Autodesk Inventor part; units mm, degrees
ref_plane "Work Plane1" through (1.525, 0, 0) normal (0, 0, 1) x (1, 0, 0)
ref_plane "YZ Plane" through (0, 0, 0) normal (1, 0, 0) x (0, 1, 0)
ref_plane "XZ Plane" through (0, 0, 0) normal (0, 1, 0) x (-1, 0, 0)
sketch "Sketch1" plane through (0, 0, 0) normal (0, 0, 1) x (1, 0, 0)
  line L0 (0, 3.175) -> (38.1, 3.175)
  line L1 (38.1, 3.175) -> (38.1, 0)
  line L2 (38.1, 0) -> (0, 0)
  line L3 (-7.62, 0) -> (45.72, 0)
  line L4 (0, -0.635) -> (0, 3.81)
  line L5 (0, 3.175) -> (0, 0)
  dimension "d2" = 6.35
  dimension "d59" = 38.1
revolve "Body" add sketch "Sketch1" angle 360 about axis through (38.1, 0, 0) along (-1, 0, 0)
sketch "Sketch2" plane through (0, 0, 0) normal (-1, 0, 0) x (0, 0, 1)
  line L0 (0, 6.4231) -> (5.5626, 3.2116)
  line L1 (5.5626, 3.2116) -> (5.5626, -3.2116)
  line L2 (5.5626, -3.2116) -> (0, -6.4231)
  line L3 (0, -6.4231) -> (-5.5626, -3.2116)
  line L4 (-5.5626, -3.2116) -> (-5.5626, 3.2116)
  line L5 (-5.5626, 3.2116) -> (0, 6.4231)
  line L6 (-7.7876, 0) -> (7.7876, 0)
  line L7 (0, 8.9924) -> (0, -8.9924)
  point P0 (0, 0)
  point P1 (0, 0)
  dimension "d11" = 11.1252
extrude "Head" add sketch "Sketch2" along normal blind 4.826
sketch "Sketch4" plane through (0, 0, 0) normal (0, 0, 1) x (1, 0, 0)
  line L0 (-4.1837, 6.6751) -> (-4.826, 5.5626)
  line L1 (-1.1, 0) -> (-0.234, 0)
  line L2 (-5.7444, 0) -> (0.6844, 0)
  line L3 (-4.826, 6.6751) -> (-4.1837, 6.6751)
  line L4 (-4.826, 5.5626) -> (-4.826, 6.6751)
  line L5 (0, 8.0101) -> (0, -1.335)
  dimension "d65" = 11.1252
  dimension "d67" = 30
  dimension "d68" = 13.3502
  dimension "d69" = 4.826
revolve "Chamfer1" cut sketch "Sketch4" angle 360 about axis through (-1.1, 0, 0) along (1, 0, 0)
thread "Thread"
chamfer "Chamfer2" distance 0.635 distance2 0.6351 1 edges at (38.1, -3.175, 0) measured on face at (38.1, -0.8017, 1.6073)
fillet "Fillet" radius 0.0635 1 edges at (0, -3.175, 0)
ref_plane "Work Plane1" through (1.525, 0, 0) normal (0, 0, 1) x (1, 0, 0)
equation "\"d2\" = GD"
equation "\"d59\" = NLG"
equation "\"d11\" = SW"
equation "\"d3\" = KOH"
equation "\"d15\" = GEL"
equation "\"d6\" = -0.5 * SPD + 0.5 * GD"
equation "\"d71\" = RR"
equation "\"d65\" = SW"
equation "\"d67\" = ANG1"
equation "\"d68\" = 1.2 * SW"
equation "\"d69\" = KOH"
equation "\"NLG\" = 38.1"
equation "\"GD\" = NND"
equation "\"BDM\" = NND"
equation "\"KOH\" = 4.826"
equation "\"GEL\" = 32.385"
equation "\"SW\" = 11.1252"
equation "\"SW0\" = SW"
equation "\"SPD\" = GD1"
equation "\"SD2\" = NND"
equation "\"SD\" = 0"
equation "\"ANG1\" = 30deg"
equation "\"GAL\" = 0.635"
equation "\"GUL\" = GAL"
equation "\"RR\" = 0.0635"
equation "\"RR1\" = 0.1"
equation "\"GD1\" = 5.08"
equation "\"THREADDIA\" = 6.35"
equation "\"SDH\" = SW"
equation "\"TOA\" = 30deg"
equation "\"NND\" = 6.35"
equation "\"E0\" = 1.155 * SW"
properties part number "ANSI B18.6.3 - 1/4-20 UNC - 1.5" material "Steel, Mild"
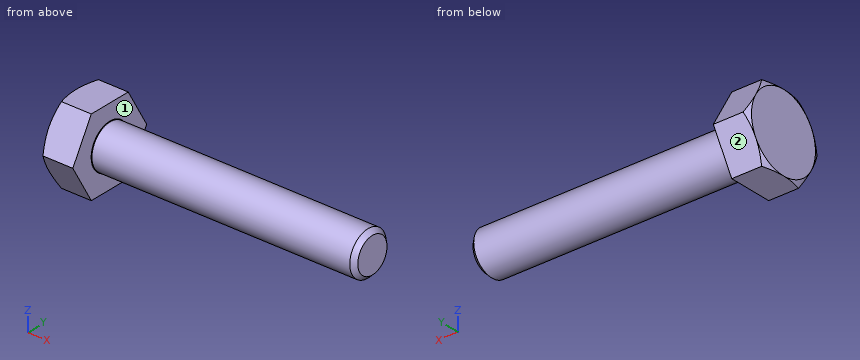
Could you check a few things on this model? Use its own coordinates, in mm. Face numbers are marked on the shaded views. A direction names the side the tool comes from. Coordinates: 2 decimals unless noted, no trailing zeros. Order: outer loops, then holes, each group sorted by start corner. A loop starts at its lowest first (then second) coordinate and runs counter-clockwise, first axis right, second up. Notation, with made-up numbers: (-1.5, 9.25) - (43.5, 9.25) arc R18 ccw to (43.5, 33.25) - close; hole circle Ø7 at (16, -22). An arc over 180 degrees is marked (long way). Answer in a Markdown table with one row per item. Add a question column.
(1) If we section it at A-A, the plane x = 16: Please give me the cut outline in (y, z) (3 decimals), then the cut area to 3 significant figures.
(2) On a 3-axis mill with a long thin cutter (end or side, diameter ignored), from which of +Z, -Z, +X, -X, +Y, -Y can I reach the whole of each face in a straight line? I mean the marked faces 1 and 2. Say none if no direction works.
(3) Will these pins go through, and if not, where does the flat tip stop? pin 1 (6 mm diameter, centred on x = 22, z = 4.5, fed in from -Y); pin 2 (1.5 mm diameter, centred on x = 32.5, z = 3.5, fed in from -Y); pin 3 (1 mm diameter, centred on x = 7.5, z = -3, fed in from -Y); pin 4 (3 mm diameter, centred on x = 8, y = -5, fed in from -Z).
(4) I need wall thicknesses on L1, parallel to X at y = -3.75, z = -1.5; L2, parallel to Z at x = 7, y = 1; L3, parallel to Z at x = 22, y = -0.25. Which ranges of each line are inside material? Lowest first, please.
Results are:
| question | item | result |
|---|---|---|
| 1 | outline | circle Ø6.35 at (0, 0) |
| 1 | area | 31.7 mm2 |
| 2 | face 1 | +X |
| 2 | face 2 | -Z, +X, -X, +Y |
| 3 | pin 1 | stops at y = -2.8 |
| 3 | pin 2 | stops at y = -1.59 |
| 3 | pin 3 | stops at y = -1.96 |
| 3 | pin 4 | passes through |
| 4 | L1 | x = -4.83 to 0 |
| 4 | L2 | z = -3.01 to 3.01 |
| 4 | L3 | z = -3.17 to 3.17 |
